Here's how the part is built. I have some questions about the finished solid (model axes, mm). Give positions to 0.01 mm unless a question says otherwise; leave off trailing zeros. Write each loop counter-clockwise with the first axis right and the second up, starting at its lowest first coordinate (ties: lowest second). Pieces come first, ordered by that corner, then holes. Notation, with made-up numbers: M 16.25,47.5 L 20.25,47.5 A16 ccw 20.25,70.5 Z; hole C 17.25,-15 d9. An arc over 180 degrees is marked long. Answer as CSV lines item,"result". Start each with the question number.
Q1. Suppose I cut it at D-D (y = 13). Write out the boundary of the cut face in (x, z).
Q2. If I drill on line 1 along X through (y, z) = (1.5, 2.6); line 2 along X through (y, z) = (-3.5, 3.25); line 3 along Y through (x, z) = (1, 3.65), over which ranges is the centre line in solid material (lowest first)?
Q3. Suppose I cut it at C-C (y = 4.5). Write out the boundary of the cut face in (x, z).
Q4. For pin 1 (1.5 mm diameter, centred on y = -8.5, z = 0.5, fed in from -X), with a flat end and sliding along its axis, tell me the tip position at first contact or that it passes through.
Q5. Suppose I cut it at B-B (x = -1.5). Write out the boundary of the cut face in (y, z).
Q6. Suppose I cut it at A-A (z = 1.7). Write out the boundary of the cut face in (x, y), then the cut area to 3 significant figures.
Q7. Thinking about a two-plate mould opening in X: for faces 1 (the flat face through (-16.93, 2.93, 2.46)), 2 (the cylindrical face through (-7.493, 0.33, 2.535)), 3 (the flat face through (16.93, -2.93, 2.46)), which applies, +X half, -X half, draft (parallel to the pull), parting line (faces both ways), or undercut?
```python
from build123d import *

# Parameters (mm, degrees)
F1_DEPTH = 5
F2_R     = 7.5
F3_DEPTH = 25


with BuildPart() as f1:
    # F0 (on Top) → F1 (new body)
    with BuildSketch(Plane.XY):
        with BuildLine():
            ThreePointArc((13.93824703, 5.5430379513), (14.7321706726, 2.8219049018), (15, 0))
            ThreePointArc((15, 0), (14.7321706726, -2.8219049018), (13.93824703, -5.5430379513))
            Line((13.93824703, -5.5430379513), (13.9437634587, -5.7756959351))
            Line((13.9437634587, -5.7756959351), (20, 0))
            Line((20, 0), (13.9437634587, 5.7756959351))
            Line((13.9437634587, 5.7756959351), (13.93824703, 5.5430379513))
        make_face()
        with BuildLine():
            ThreePointArc((13.7753487165, 5.9363092691), (13.8581929877, 5.7402514855), (13.93824703, 5.5430379513))
            Line((13.93824703, 5.5430379513), (13.9437634587, 5.7756959351))
            Line((13.9437634587, 5.7756959351), (13.7753487165, 5.9363092691))
        make_face()
        with BuildLine():
            Line((13.9437634587, -5.7756959351), (13.93824703, -5.5430379513))
            ThreePointArc((13.93824703, -5.5430379513), (13.8581929877, -5.7402514855), (13.7753487165, -5.9363092691))
            Line((13.7753487165, -5.9363092691), (13.9437634587, -5.7756959351))
        make_face()
        with BuildLine():
            ThreePointArc((5.9363092691, 13.7753487165), (10.6066017178, 10.6066017178), (13.7753487165, 5.9363092691))
            Line((13.7753487165, 5.9363092691), (13.9437634587, 5.7756959351))
            Line((13.9437634587, 5.7756959351), (14.1421356237, 14.1421356237))
            Line((14.1421356237, 14.1421356237), (5.7756959351, 13.9437634587))
            Line((5.7756959351, 13.9437634587), (5.9363092691, 13.7753487165))
        make_face()
        with BuildLine():
            Line((13.9437634587, -5.7756959351), (13.7753487165, -5.9363092691))
            ThreePointArc((13.7753487165, -5.9363092691), (10.6066017178, -10.6066017178), (5.9363092691, -13.7753487165))
            Line((5.9363092691, -13.7753487165), (5.7756959351, -13.9437634587))
            Line((5.7756959351, -13.9437634587), (14.1421356237, -14.1421356237))
            Line((14.1421356237, -14.1421356237), (13.9437634587, -5.7756959351))
        make_face()
        with BuildLine():
            ThreePointArc((5.5430379513, 13.93824703), (5.7402514855, 13.8581929877), (5.9363092691, 13.7753487165))
            Line((5.9363092691, 13.7753487165), (5.7756959351, 13.9437634587))
            Line((5.7756959351, 13.9437634587), (5.5430379513, 13.93824703))
        make_face()
        with BuildLine():
            Line((5.7756959351, -13.9437634587), (5.9363092691, -13.7753487165))
            ThreePointArc((5.9363092691, -13.7753487165), (5.7402514855, -13.8581929877), (5.5430379513, -13.93824703))
            Line((5.5430379513, -13.93824703), (5.7756959351, -13.9437634587))
        make_face()
        with BuildLine():
            ThreePointArc((0, 15), (2.8219049018, 14.7321706726), (5.5430379513, 13.93824703))
            Line((5.5430379513, 13.93824703), (5.7756959351, 13.9437634587))
            Line((5.7756959351, 13.9437634587), (0, 20))
            Line((0, 20), (0, 15))
        make_face()
        with BuildLine():
            Line((5.7756959351, -13.9437634587), (5.5430379513, -13.93824703))
            ThreePointArc((5.5430379513, -13.93824703), (0, -15), (-5.5430379513, -13.93824703))
            Line((-5.5430379513, -13.93824703), (-5.7756959351, -13.9437634587))
            Line((-5.7756959351, -13.9437634587), (0, -20))
            Line((0, -20), (5.7756959351, -13.9437634587))
        make_face()
        with BuildLine():
            ThreePointArc((-5.5430379513, 13.93824703), (-2.8219049018, 14.7321706726), (0, 15))
            Line((0, 15), (0, 20))
            Line((0, 20), (-5.7756959351, 13.9437634587))
            Line((-5.7756959351, 13.9437634587), (-5.5430379513, 13.93824703))
        make_face()
        with BuildLine():
            Line((-5.7756959351, -13.9437634587), (-5.5430379513, -13.93824703))
            ThreePointArc((-5.5430379513, -13.93824703), (-5.7402514855, -13.8581929877), (-5.9363092691, -13.7753487165))
            Line((-5.9363092691, -13.7753487165), (-5.7756959351, -13.9437634587))
        make_face()
        with BuildLine():
            ThreePointArc((-5.9363092691, 13.7753487165), (-5.7402514855, 13.8581929877), (-5.5430379513, 13.93824703))
            Line((-5.5430379513, 13.93824703), (-5.7756959351, 13.9437634587))
            Line((-5.7756959351, 13.9437634587), (-5.9363092691, 13.7753487165))
        make_face()
        with BuildLine():
            Line((-5.9363092691, 13.7753487165), (-5.7756959351, 13.9437634587))
            Line((-5.7756959351, 13.9437634587), (-14.1421356237, 14.1421356237))
            Line((-14.1421356237, 14.1421356237), (-13.9437634587, 5.7756959351))
            Line((-13.9437634587, 5.7756959351), (-13.7753487165, 5.9363092691))
            ThreePointArc((-13.7753487165, 5.9363092691), (-10.6066017178, 10.6066017178), (-5.9363092691, 13.7753487165))
        make_face()
        with BuildLine():
            Line((-5.7756959351, -13.9437634587), (-5.9363092691, -13.7753487165))
            ThreePointArc((-5.9363092691, -13.7753487165), (-10.6066017178, -10.6066017178), (-13.7753487165, -5.9363092691))
            Line((-13.7753487165, -5.9363092691), (-13.9437634587, -5.7756959351))
            Line((-13.9437634587, -5.7756959351), (-14.1421356237, -14.1421356237))
            Line((-14.1421356237, -14.1421356237), (-5.7756959351, -13.9437634587))
        make_face()
        with BuildLine():
            Line((-13.9437634587, -5.7756959351), (-13.7753487165, -5.9363092691))
            ThreePointArc((-13.7753487165, -5.9363092691), (-13.8581929877, -5.7402514855), (-13.93824703, -5.5430379513))
            Line((-13.93824703, -5.5430379513), (-13.9437634587, -5.7756959351))
        make_face()
        with BuildLine():
            ThreePointArc((-13.93824703, 5.5430379513), (-13.8581929877, 5.7402514855), (-13.7753487165, 5.9363092691))
            Line((-13.7753487165, 5.9363092691), (-13.9437634587, 5.7756959351))
            Line((-13.9437634587, 5.7756959351), (-13.93824703, 5.5430379513))
        make_face()
        with BuildLine():
            Line((-13.93824703, 5.5430379513), (-13.9437634587, 5.7756959351))
            Line((-13.9437634587, 5.7756959351), (-20, 0))
            Line((-20, 0), (-13.9437634587, -5.7756959351))
            Line((-13.9437634587, -5.7756959351), (-13.93824703, -5.5430379513))
            ThreePointArc((-13.93824703, -5.5430379513), (-15, 0), (-13.93824703, 5.5430379513))
        make_face()
        with BuildLine():
            ThreePointArc((13.93824703, -5.5430379513), (14.7321706726, -2.8219049018), (15, 0))
            ThreePointArc((15, 0), (14.7321706726, 2.8219049018), (13.93824703, 5.5430379513))
            ThreePointArc((13.93824703, 5.5430379513), (13.8581929877, 5.7402514855), (13.7753487165, 5.9363092691))
            ThreePointArc((13.7753487165, 5.9363092691), (10.6066017178, 10.6066017178), (5.9363092691, 13.7753487165))
            ThreePointArc((5.9363092691, 13.7753487165), (5.7402514855, 13.8581929877), (5.5430379513, 13.93824703))
            ThreePointArc((5.5430379513, 13.93824703), (2.8219049018, 14.7321706726), (0, 15))
            ThreePointArc((0, 15), (-2.8219049018, 14.7321706726), (-5.5430379513, 13.93824703))
            ThreePointArc((-5.5430379513, 13.93824703), (-5.7402514855, 13.8581929877), (-5.9363092691, 13.7753487165))
            ThreePointArc((-5.9363092691, 13.7753487165), (-10.6066017178, 10.6066017178), (-13.7753487165, 5.9363092691))
            ThreePointArc((-13.7753487165, 5.9363092691), (-13.8581929877, 5.7402514855), (-13.93824703, 5.5430379513))
            ThreePointArc((-13.93824703, 5.5430379513), (-15, 0), (-13.93824703, -5.5430379513))
            ThreePointArc((-13.93824703, -5.5430379513), (-13.8581929877, -5.7402514855), (-13.7753487165, -5.9363092691))
            ThreePointArc((-13.7753487165, -5.9363092691), (-10.6066017178, -10.6066017178), (-5.9363092691, -13.7753487165))
            ThreePointArc((-5.9363092691, -13.7753487165), (-5.7402514855, -13.8581929877), (-5.5430379513, -13.93824703))
            ThreePointArc((-5.5430379513, -13.93824703), (0, -15), (5.5430379513, -13.93824703))
            ThreePointArc((5.5430379513, -13.93824703), (5.7402514855, -13.8581929877), (5.9363092691, -13.7753487165))
            ThreePointArc((5.9363092691, -13.7753487165), (10.6066017178, -10.6066017178), (13.7753487165, -5.9363092691))
            ThreePointArc((13.7753487165, -5.9363092691), (13.8581929877, -5.7402514855), (13.93824703, -5.5430379513))
        make_face()
    extrude(amount=F1_DEPTH)

    # F2 (on face) → F3 (cut)
    with BuildSketch(Plane.XY.offset(5)):
        Circle(F2_R)
    extrude(amount=-F3_DEPTH, mode=Mode.SUBTRACT)


solid = f1.part
```
Resolved:
1,outline,"M -14.12,0 L 14.12,0 L 14.12,5 L -14.12,5 Z"
2,line 1,"-18.43 to -7.35, 7.35 to 18.43"
2,line 2,"-16.33 to -6.63, 6.63 to 16.33"
2,line 3,"-18.95 to -7.43, 7.43 to 18.95"
3,outline,"M -15.28,0 L -6,0 L -6,5 L -15.28,5 Z; M 6,0 L 15.28,0 L 15.28,5 L 6,5 Z"
4,pin 1,"x = -14.03"
5,outline,"M -18.43,0 L -7.35,0 L -7.35,5 L -18.43,5 Z; M 7.35,0 L 18.43,0 L 18.43,5 L 7.35,5 Z"
6,outline,"M -20,0 L -13.94,-5.78 L -14.14,-14.14 L -5.78,-13.94 L 0,-20 L 5.78,-13.94 L 14.14,-14.14 L 13.94,-5.78 L 20,0 L 13.94,5.78 L 14.14,14.14 L 5.78,13.94 L 0,20 L -5.78,13.94 L -14.14,14.14 L -13.94,5.78 Z; hole C 0,0 d15"
6,area,"747 mm^2"
7,face 1,"-X half"
7,face 2,"undercut"
7,face 3,"+X half"
